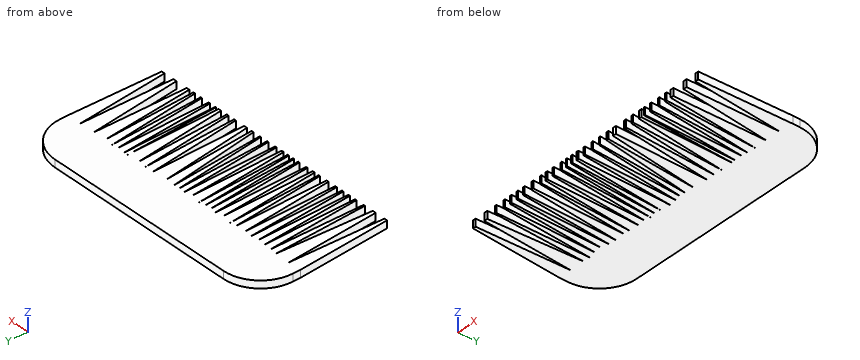
from build123d import *

# Parameters (mm, degrees)
F1_DEPTH = 2.54
F2_R     = 12.7


with BuildPart() as f1:
    # F0 (on Top) → F1 (new body)
    with BuildSketch(Plane.XY):
        Polygon((73.3829085314, 9.4430754296), (-18.0570914686, 9.4430754296), (-18.0570914686, -5.7969245704), (-13.6215174571, -5.7969245704), (-8.4692621604, -5.7969245704), (-6.0992240906, -5.7969245704), (-3.5184609428, -5.7969245704), (-0.937697795, -5.7969245704), (1.6430653527, -5.7969245704), (4.2052869685, -5.7969245704), (7.6057757251, -5.7969245704), (9.6666784957, -5.7969245704), (13.0671672523, -5.7969245704), (15.6479304001, -5.7969245704), (17.7088331707, -5.7969245704), (19.7697359413, -5.7969245704), (21.8306387119, -5.7969245704), (25.2311274685, -5.7969245704), (27.8118906163, -5.7969245704), (29.8727933869, -5.7969245704), (31.816742076, -5.7969245704), (35.011141254, -5.7969245704), (39.9619415402, -5.7969245704), (42.8472035564, -5.7969245704), (45.7324655727, -5.7969245704), (49.9573135749, -5.7969245704), (51.2968995608, -5.7969245704), (53.8776627086, -5.7969245704), (55.9385654792, -5.7969245704), (58.8238274954, -5.7969245704), (63.2547683358, -5.7969245704), (68.5100684218, -5.7969245704), (73.3829085314, -5.7969245704), align=None)
        Polygon((-13.6215174571, -5.7969245704), (-18.0570914686, -5.7969245704), (-16.0638535681, -37.1604112962), (-15.0540701944, -37.1604112962), align=None)
        Polygon((-8.4692621604, -5.7969245704), (-13.6215174571, -5.7969245704), (-11.6282795566, -37.1604112962), (-10.455339657, -37.1604112962), align=None)
        Polygon((-6.0992240906, -5.7969245704), (-8.4692621604, -5.7969245704), (-7.4346404592, -37.1604112962), (-6.8950879612, -37.1604112962), align=None)
        Polygon((-3.5184609428, -5.7969245704), (-6.0992240906, -5.7969245704), (-4.1059861901, -37.1604112962), (-3.5184609428, -37.1604112962), align=None)
        Polygon((-0.937697795, -5.7969245704), (-3.5184609428, -5.7969245704), (-1.5252230424, -37.1604112962), (-0.937697795, -37.1604112962), align=None)
        Polygon((1.6430653527, -5.7969245704), (-0.937697795, -5.7969245704), (1.0555401054, -37.1604112962), (1.6430653527, -37.1604112962), align=None)
        Polygon((4.2052869685, -5.7969245704), (1.6430653527, -5.7969245704), (3.6320772404, -37.1604112962), (4.2052869685, -37.1604112962), align=None)
        Polygon((7.6057757251, -5.7969245704), (4.2052869685, -5.7969245704), (6.831635332, -37.1604112962), (7.6057757251, -37.1604112962), align=None)
        Polygon((13.0671672523, -5.7969245704), (9.6666784957, -5.7969245704), (12.2930268592, -37.1604112962), (13.0671672523, -37.1604112962), align=None)
        Polygon((15.6479304001, -5.7969245704), (13.0671672523, -5.7969245704), (15.0604051528, -37.1604112962), (15.6479304001, -37.1604112962), align=None)
        Polygon((17.7088331707, -5.7969245704), (15.6479304001, -5.7969245704), (18.2742787636, -37.1604112962), (18.7434548718, -37.1604112962), align=None)
        Polygon((19.7697359413, -5.7969245704), (17.7088331707, -5.7969245704), (20.3351815342, -37.1604112962), (20.8043576424, -37.1604112962), align=None)
        Polygon((21.8306387119, -5.7969245704), (19.7697359413, -5.7969245704), (22.3960843048, -37.1604112962), (22.865260413, -37.1604112962), align=None)
        Polygon((30.907415088, -37.1604112962), (29.8727933869, -5.7969245704), (27.8118906163, -5.7969245704), (30.4382389798, -37.1604112962), align=None)
        Polygon((33.8099799764, -37.1604112962), (31.816742076, -5.7969245704), (29.8727933869, -5.7969245704), (33.3674291227, -37.1604112962), align=None)
        Polygon((37.0043791545, -37.1604112962), (35.011141254, -5.7969245704), (31.816742076, -5.7969245704), (36.2771562132, -37.1604112962), align=None)
        Polygon((39.9619415402, -37.1604112962), (39.9619415402, -5.7969245704), (35.011141254, -5.7969245704), (38.834864007, -37.1604112962), align=None)
        Polygon((25.2311274685, -5.7969245704), (21.8306387119, -5.7969245704), (24.4569870754, -37.1604112962), (25.2311274685, -37.1604112962), align=None)
        Polygon((27.8118906163, -37.1604112962), (27.8118906163, -5.7969245704), (25.2311274685, -5.7969245704), (27.2243653689, -37.1604112962), align=None)
        Polygon((43.8818252576, -37.1604112962), (42.8472035564, -5.7969245704), (39.9619415402, -5.7969245704), (43.2249791301, -37.1604112962), align=None)
        Polygon((46.7670872738, -37.1604112962), (45.7324655727, -5.7969245704), (42.8472035564, -5.7969245704), (46.1102411463, -37.1604112962), align=None)
        Polygon((49.9573135749, -37.1604112962), (49.9573135749, -5.7969245704), (45.7324655727, -5.7969245704), (48.9955031625, -37.1604112962), align=None)
        Polygon((51.2968995608, -37.1604112962), (51.2968995608, -5.7969245704), (49.9573135749, -5.7969245704), (50.991935276, -37.1604112962), align=None)
        Polygon((53.8776627086, -37.1604112962), (53.8776627086, -5.7969245704), (51.2968995608, -5.7969245704), (53.2901374613, -37.1604112962), align=None)
        Polygon((56.9731871804, -37.1604112962), (55.9385654792, -5.7969245704), (53.8776627086, -5.7969245704), (56.5040110721, -37.1604112962), align=None)
        Polygon((59.8584491966, -37.1604112962), (58.8238274954, -5.7969245704), (55.9385654792, -5.7969245704), (59.201603069, -37.1604112962), align=None)
        Polygon((62.4589044652, -37.1604112962), (63.2547683358, -5.7969245704), (58.8238274954, -5.7969245704), (61.4501758589, -37.1604112962), align=None)
        Polygon((67.7142045512, -37.1604112962), (68.5100684218, -5.7969245704), (63.2547683358, -5.7969245704), (66.5178059256, -37.1604112962), align=None)
        Polygon((72.2457462459, -37.1604112962), (73.3829085314, -5.7969245704), (68.5100684218, -5.7969245704), (71.1364167853, -37.1604112962), align=None)
        Polygon((9.6666784957, -5.7969245704), (7.6057757251, -5.7969245704), (10.2321240886, -37.1604112962), (10.7013001968, -37.1604112962), align=None)
    extrude(amount=F1_DEPTH)

    # F2
    f2_edges = [f1.edges().sort_by_distance(p)[0] for p in [
        (73.382909, 9.443075, 1.27),
        (-18.057091, 9.443075, 1.27),
    ]]
    fillet(f2_edges, radius=F2_R)


solid = f1.part
Read the model definition and answer for the solid it produces. Units are mm, in the model's axes. Round coordinates to 2 decimals unless told otherwise and drop trailing zeros. Write each loop counter-clockwise with the first axis right and the second up, starting at its lowest first coordinate (ties: lowest second). Pieces come first, ordered by that corner, then holes. Notation, with made-up numbers: (-18.5, -15.75) - (32.5, -15.75) arc R30 cw to (32.5, 12.25) - close; hole circle Ø9 at (17, 12.5). An arc over 180 degrees is marked (long way). Use a Markdown table: item, result.
(1) Each of these flat-tipped pins is pushed along its axis until it touches: pin 1 Ø1.3 at (y, z) = (-20, 1) entering from +X; pin 2 Ø0.8 at (y, z) = (-22.5, 0.5) entering from +X; pin 3 Ø1.3 at (y, z) = (-28, 1.5) entering from +X. Where does it stop, or does it pass through?
Reported:
| item | result |
|---|---|
| pin 1 | x = 72.89 |
| pin 2 | x = 72.79 |
| pin 3 | x = 72.6 |
(2) The part is cut by section B-B (x = 6). Write down the section's boundary in (y, z), then the cut area to 3 significant figures.
Reported:
| item | result |
|---|---|
| outline | (-27.23, 0) - (9.44, 0) - (9.44, 2.54) - (-27.23, 2.54) - close |
| area | 93.1 mm2 |
(3) Straight lines are drawn through the part: line 1 along X through (y, z) = (-3, 2.05); line 2 along X through (y, z) = (-1, 1.8). For each, find the intervals that lie inside material, in ascending order. Write a range as [from, to].
Reported:
| item | result |
|---|---|
| line 1 | [-18.05, 73.38] |
| line 2 | [-17.85, 73.18] |
(4) The part is cut by section A-A (y = -23.5). State how many separate pieces and enclosed holes the cut face has, then the cut area to 3 significant figures.
Reported:
| item | result |
|---|---|
| separate pieces | 30 |
| enclosed holes | 0 |
| area | 131 mm2 |
(5) The part is cut by section D-D (x = 29). Write down the section's boundary in (y, z), then the cut area to 3 significant figures.
Reported:
| item | result |
|---|---|
| outline | (-19.99, 0) - (9.44, 0) - (9.44, 2.54) - (-19.99, 2.54) - close |
| area | 74.7 mm2 |
